Geometry check sheet. Reference: drawing and pictorial views, mm from the part's lowest x, y, z. Round coordinates to 2 decimals unless told otherwise and drop trailing zeros. Loops run counter-clockwise (first coordinate to the right, second up) from the corner with the lowest first, then second, coordinate; pieces in that order, holes last. Notation, with made-up numbers: (22.25, 62.25) -> (70.25, 62.25) arc R27 cw to (70.25, 95.25) -> close; hole circle Ø2 at (81.25, 48). An arc over 180 degrees is marked (long way). Use one line per item in the form item = value.
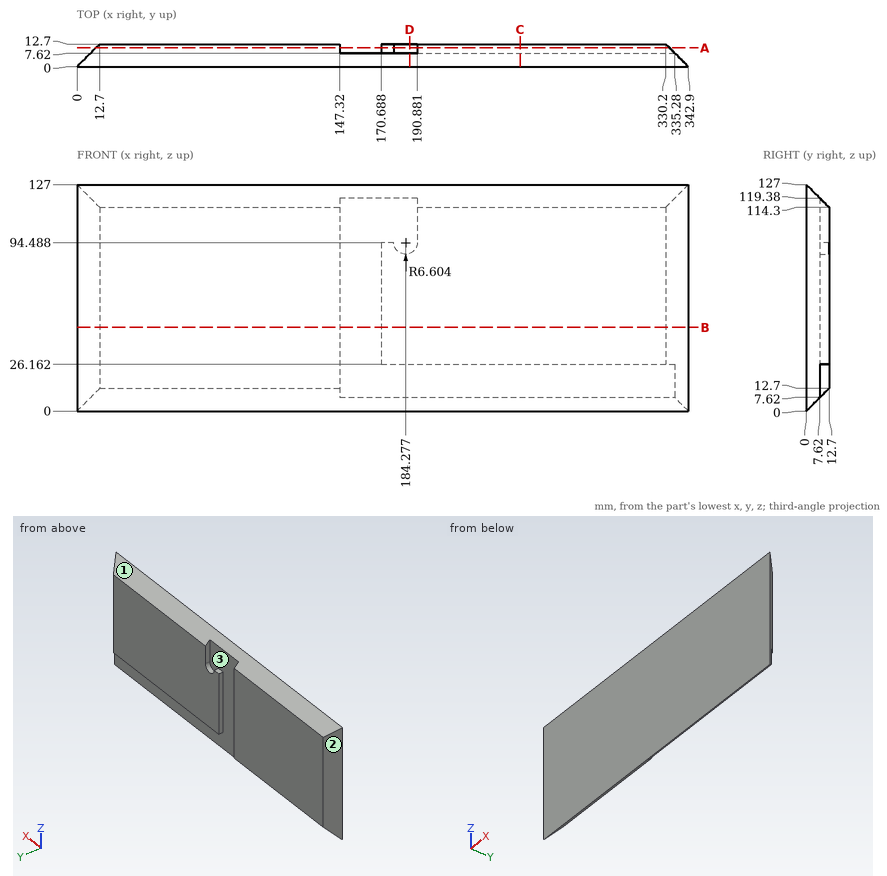
1. Gauge pin test, flat ends, axial feed: pin 1 (2.5 mm diameter, centred on y = 10.5, z = 57, fed in from -X); pin 2 (1.5 mm diameter, centred on y = 7, z = 98, fed in from -X); pin 3 (6 mm diameter, centred on y = 6.5, z = 65.5, fed in from -X). Record the tip position at first contact, or that the pin passes through.
Return value:
pin_1 = 9.25
pin_2 = 6.25
pin_3 = 3.5
2. Section check C-C (x = 248.5). Record the boundary of the cut face in (y, z), then the cut area to 3 significant figures.
Return value:
outline = (0, 0) -> (7.62, 7.62) -> (7.62, 26.16) -> (12.7, 26.16) -> (12.7, 114.3) -> (0, 127) -> close
area = 1,370 mm2
3. Section check D-D (x = 186.5). Record the boundary of the cut face in (y, z).
Return value:
outline = (0, 0) -> (7.62, 7.62) -> (7.62, 26.16) -> (12.7, 26.16) -> (12.7, 88.27) -> (7.62, 88.27) -> (7.62, 119.38) -> (0, 127) -> close
4. Material ranges on line 1 along X through (y, z) = (9.25, 89); line 2 along Y through (x, z) = (218.5, 16); line 3 along Z through (x, y) = (54, 5.5), recorded low to high.
Return value:
line_1 = 9.25 to 147.32, 170.69 to 180.6, 187.95 to 333.65
line_2 = 0 to 7.62
line_3 = 5.5 to 121.5
5. Section check B-B (z = 47). Record the boundary of the cut face in (x, y).
Return value:
outline = (0, 0) -> (342.9, 0) -> (330.2, 12.7) -> (170.69, 12.7) -> (170.69, 7.62) -> (147.32, 7.62) -> (147.32, 12.7) -> (12.7, 12.7) -> close
6. Section check A-A (y = 10.5). Record the boundary of the cut face in (x, z).
Return value:
outline = (10.5, 10.5) -> (147.32, 10.5) -> (147.32, 116.5) -> (10.5, 116.5) -> close; (170.69, 26.16) -> (332.4, 26.16) -> (332.4, 116.5) -> (190.88, 116.5) -> (190.88, 94.49) arc R6.6 cw to (177.67, 94.49) -> (170.69, 94.49) -> close
7. Mould release check, pull along X, two halves, no side actions. Record for the marked faces 1, 2 and 3: released by +X, released by -X, zero draft, split by the parting line, or undercut.
Return value:
face_1 = zero draft
face_2 = released by -X
face_3 = undercut
